Here's how the part is built. I have some questions about the finished solid (model axes, mm). A direction names the side the tool comes from. Give positions to 0.01 mm unless a question says otherwise; leave off trailing zeros. Loops run counter-clockwise (first coordinate to the right, second up) from the corner with the lowest first, then second, coordinate; pieces in that order, holes last.
Q1. I'm going to push a flat-ended pin straight in: P1, Ø0.8, axis at x = -71.5, y = 11.5, coming from the -Z side. Where does the tip first touch, or does it pass through?
Q2. Suppose I cut it at A-A (z = -142). List the corners of the cut face in (x, y) for me, and give its area (3 significant figures).
Q3. I need wall thicknesses on probe 1 along X at (y, z) = (4.75, -89); probe 2 along X at (y, z) = (11.5, -55.5); probe 3 along Z at (x, y) = (49, 2.5). Which ranges of each line are inside material? Lowest first, please.
Q4. Thinking about a two-plate mould opening in Y: for faces 1 (the face through (-1, 0, -2)), 2 (the face through (171, 6, -93)), 3 (the face through (26, 1, -4)), which applies, pulls with the +Y half, pulls with the -Y half, needs draft (parallel to the pull), parting line crosses it, or undercut?
Q5. For faces 4 (the face through (-171, 6, -96)), 5 (the face through (170, 6, -97)), which set-ups out of +Z, -Z, +X, -X, +Y, -Y let a thin tool reach every point of the face, with its end or its side?
Q6. Suppose I cut it at C-C (x = -54.5). List the corners of the cut face in (y, z) for me.
Q7. Suppose I cut it at B-B (y = 9). List the corners of the cut face in (x, z) for me, and give its area (3 significant figures).
```python
from build123d import *

# Parameters (mm, degrees)
CROQUIS2_W              = 342
CROQUIS2_H              = 20
CROQUIS2_W_2            = 20
CROQUIS2_H_2            = 189.712394883
SALIENTE_EXTRUIR2_DEPTH = 12
CROQUIS3_W              = 340
CROQUIS3_H              = 10
CORTAR_EXTRUIR1_DEPTH   = 208


with BuildPart() as part:
    # Croquis2 → Saliente-Extruir2 (new body)
    with BuildSketch(Plane(origin=(0, 0, 0), x_dir=(1, 0, 0), z_dir=(0, 1, 0))):
        Rectangle(CROQUIS2_W, CROQUIS2_H)
        with Locations((161, 104.856197442)):
            Rectangle(CROQUIS2_W_2, CROQUIS2_H_2)
        with Locations((-161, 104.856197442)):
            Rectangle(CROQUIS2_W_2, CROQUIS2_H_2)
    extrude(amount=SALIENTE_EXTRUIR2_DEPTH)

    # Croquis3 → Cortar-Extruir1 (cut)
    with BuildSketch(Plane(origin=(0, 0, -199.712394883), x_dir=(-1, 0, 0), z_dir=(0, 0, -1))):
        with Locations((0, 6)):
            Rectangle(CROQUIS3_W, CROQUIS3_H)
    extrude(amount=-CORTAR_EXTRUIR1_DEPTH, mode=Mode.SUBTRACT)


solid = part.part
```
Solutions:
1. P1: stops at z = -10
2. outline: (-171, 0) - (-151, 0) - (-151, 1) - (-170, 1) - (-170, 11) - (-151, 11) - (-151, 12) - (-171, 12) - close; (151, 0) - (171, 0) - (171, 12) - (151, 12) - (151, 11) - (170, 11) - (170, 1) - (151, 1) - close
2. area: 100 mm2
3. probe 1: x = -171 to -170, 170 to 171
3. probe 2: x = -171 to -151, 151 to 171
3. probe 3: z = 8.29 to 10
4. face 1: pulls with the -Y half
4. face 2: needs draft
4. face 3: undercut
5. face 4: +Z, -Z, -X, +Y, -Y
5. face 5: -Z
6. outline: (0, -10) - (1, -10) - (1, 8.29) - (11, 8.29) - (11, -10) - (12, -10) - (12, 10) - (0, 10) - close
7. outline: (-171, -199.71) - (-170, -199.71) - (-170, 8.29) - (170, 8.29) - (170, -199.71) - (171, -199.71) - (171, 10) - (-171, 10) - close
7. area: 1,000 mm2
